from build123d import *

# Parameters (mm, degrees)
F1_DEPTH = 60
F3_W     = 12
F3_H     = 12
F4_DEPTH = 2
F5_DEPTH = 30
F6_W     = 2
F6_H     = 3
F6_H_2   = 4
F7_DEPTH = 9.501


with BuildPart() as f1:
    # F0 (on Top) → F1 (new body)
    with BuildSketch(Plane.XY):
        with BuildLine():
            Line((-9.5, 0), (-7.5, 0))
            ThreePointArc((-7.5, 0), (0, 7.5), (7.5, 0))
            Line((7.5, 0), (9.5, 0))
            Line((9.5, 0), (9.5, 9.5))
            Line((9.5, 9.5), (-9.5, 9.5))
            Line((-9.5, 9.5), (-9.5, 0))
        make_face()
    extrude(amount=-F1_DEPTH)

    # F3 (on offset) → F4 (join)
    with BuildSketch(Plane.XY.offset(-10)):
        with Locations((-13.5, 3.5)):
            Rectangle(F3_W, F3_H)
        with Locations((13.5, 3.5)):
            Rectangle(F3_W, F3_H)
    extrude(amount=F4_DEPTH)

    # F1_face (on face) → F5 (join)
    with BuildSketch(Plane(origin=(0, 6.25253, 0), x_dir=(1, 0, 0), z_dir=(0, 0, 1))):
        with BuildLine():
            Line((-9.5, -6.25253), (-7.5, -6.25253))
            ThreePointArc((-7.5, -6.25253), (0, 1.24747), (7.5, -6.25253))
            Line((7.5, -6.25253), (9.5, -6.25253))
            Line((9.5, -6.25253), (9.5, 3.24747))
            Line((9.5, 3.24747), (-9.5, 3.24747))
            Line((-9.5, 3.24747), (-9.5, -6.25253))
        make_face()
    extrude(amount=F5_DEPTH)

    # F6 (on face) → F7 (cut, through all)
    with BuildSketch(Plane.XZ):
        with Locations((-8.5, -4)):
            Rectangle(F6_W, F6_H)
        with Locations((-8.5, -56)):
            Rectangle(F6_W, F6_H)
        with Locations((8.5, -4)):
            Rectangle(F6_W, F6_H)
        with Locations((8.5, -56)):
            Rectangle(F6_W, F6_H)
        with Locations((-8.5, 25)):
            Rectangle(F6_W, F6_H_2)
        with Locations((8.5, 25)):
            Rectangle(F6_W, F6_H_2)
    extrude(amount=-F7_DEPTH, mode=Mode.SUBTRACT)


solid = f1.part
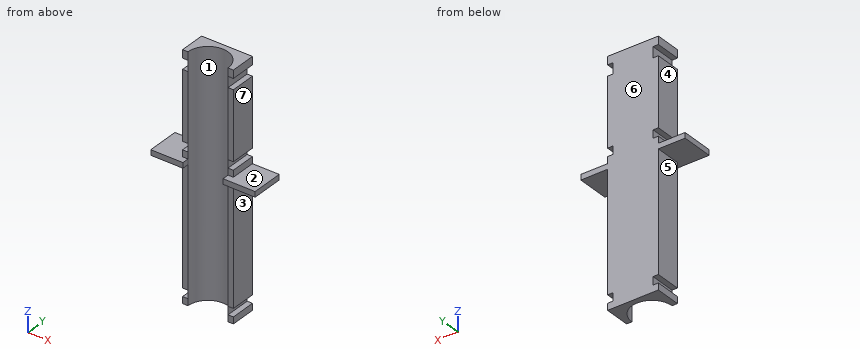
Check sheet for the modelled part. Datum: model origin and axes. Units: mm. Face numbers are marked on the shaded views. A direction names the side the tool comes from. Give positions to 0.01 mm unless a question says otherwise; leave off trailing zeros. Write each loop counter-clockwise with the first axis right and the second up, starting at its lowest first coordinate (ties: lowest second). Pieces come first, ordered by that corner, then holes. Notation, with made-up numbers: (17, 64.5) -> (42, 64.5) arc R19 ccw to (42, 89.5) -> close; hole circle Ø6 at (55, 86). An arc over 180 degrees is marked (long way). Use one line per item in the form item = value. Start each with the question number.
1. Section check A-A (z = -25). Record the cut outline in (x, y), and give its area (3 significant figures).
2. Section check B-B (x = -15). Record the cut outline in (y, z).
3. Thickness scan on line 1 along Z through (x, y) = (8.5, 5.5); line 2 along Z through (x, y) = (17, 6); line 3 along X through (y, z) = (6.75, -45.5). Record the ranges inside material, lowest first. Write a range as from..to.
4. Access from +Z, -Z, +X, -X, +Y, -Y to the whole of each face (thin tool, end or side, straight path). Record for the marked faces 4, 5, 6 and 7.
5. Go/stop test with flat-tipped pins: P1, Ø5, axis at y = 2.5, z = 11.5, coming from the -X side; P2, Ø2, axis at x = 12.5, y = 0.5, coming from the -Z side; P3, Ø3.5, axis at y = 3, z = -4, coming from the +X side. Record where each tip stops, or that it passes through.
6. Section check C-C (z = 24.5). Record the cut outline in (x, y), and give its area (3 significant figures).
7. Mould release check, pull along X, two halves, no side actions. Record for the marked faces 1, 2 and 3: pulls with the +X half, pulls with the -X half, needs draft (parallel to the pull), parting line crosses it, or undercut.
Conclusion:
q1.outline = (-9.5, 0) -> (-7.5, 0) arc R7.5 cw to (7.5, 0) -> (9.5, 0) -> (9.5, 9.5) -> (-9.5, 9.5) -> close
q1.area = 92.1 mm²
q2.outline = (-2.5, -10) -> (9.5, -10) -> (9.5, -8) -> (-2.5, -8) -> close
q3.line_1 = -60..-57.5, -54.5..-5.5, -2.5..23, 27..30
q3.line_2 = -10..-8
q3.line_3 = -9.5..-3.27, 3.27..9.5
q4.face_4 = +Z, -X, +Y, -Y
q4.face_5 = -Z, -X, +Y, -Y
q4.face_6 = +Z, -Z, +X, -X, +Y
q4.face_7 = +Z, +X, +Y, -Y
q5.P1 = -9.5
q5.P2 = -10
q5.P3 = 9.5
q6.outline = (-7.5, 0) arc R7.5 cw to (7.5, 0) -> (7.5, 9.5) -> (-7.5, 9.5) -> close
q6.area = 54.1 mm²
q7.face_1 = undercut
q7.face_2 = needs draft
q7.face_3 = pulls with the +X half
